The model under review builds one solid part; all positions refer to its coordinate system, in mm. Round coordinates to 2 decimals unless told otherwise and drop trailing zeros. Order: outer loops, then holes, each group sorted by start corner. A loop starts at its lowest first (then second) coordinate and runs counter-clockwise, first axis right, second up.
1) Consider section A-A (x = 119). Give the boundary of the cut face in (y, z), then the cut area to 3 significant figures.
2) To check wall thickness, follow L1, parallel to X at y = 7.5, z = 1177.1; L2, parallel to Y at x = 359.5, z = 911.5; L3, parallel to X at y = 13.5, z = -203.35. State the ranges of each line that lie inside material, in increasing order.
3) Consider section B-B (y = -71.5). Give the boundary of the cut face in (x, z).
4) Clearance check with flat-ended pins moving along their axes: P1, Ø7.5, axis at y = -766.5, z = 990.5, coming from the -X side; P2, Ø7.5, axis at y = 15, z = 550, coming from the +X side; P3, Ø21, axis at x = 352.21, z = -203.35, coming from the -Y side. State where each tip first meets the part, or that it passes through.
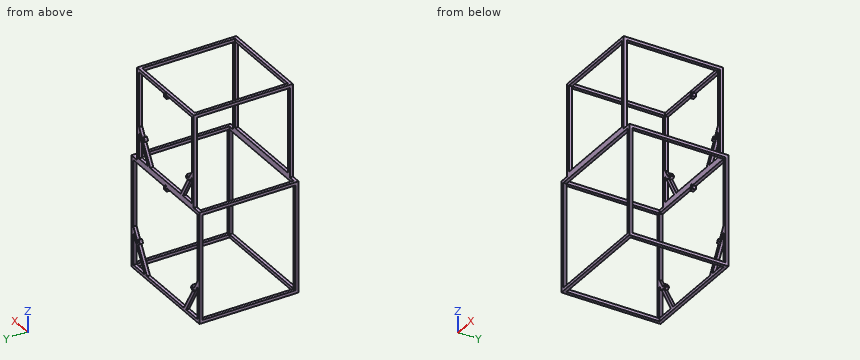
from build123d import *

# Parameters (mm, degrees)
BOSS_EXTRUDE1_DEPTH = 25
SKETCH2_R           = 6.5
CUT_EXTRUDE1_DEPTH  = 25
SKETCH3_W           = 25
SKETCH3_H           = 25
BOSS_EXTRUDE2_DEPTH = 750
SKETCH4_W           = 844.9
SKETCH4_H           = 844.9
SKETCH4_W_2         = 694.9
SKETCH4_H_2         = 694.9
BOSS_EXTRUDE3_DEPTH = 25


with BuildPart() as part:
    # Sketch1 → Boss-Extrude1 (new body)
    with BuildSketch(Plane(origin=(0, 0, 0), x_dir=(1, 0, 0), z_dir=(0, 1, 0))):
        Polygon((-447.45, -447.45), (-447.45, 447.45), (447.45, 447.45), (447.45, -447.45), (372.45, -447.45), (372.45, -1192.35), (-372.45, -1192.35), (-372.45, -447.45), align=None)
        Polygon((-422.45, 422.45), (-272.769134679, 422.45), (-422.45, 163.195136343), align=None, mode=Mode.SUBTRACT)
        Polygon((422.45, 113.195136343), (422.45, -422.45), (16, -422.45), (16, -394.45), (-16, -394.45), (-16, -422.45), (-422.45, -422.45), (-422.45, 113.195136343), (-373.852431829, 197.368593539), (-349.603720523, 183.368593539), (-333.603720523, 211.081406461), (-357.852431829, 225.081406461), (-243.901621219, 422.45), (243.901621219, 422.45), (357.852431829, 225.081406461), (333.603720523, 211.081406461), (349.603720523, 183.368593539), (373.852431829, 197.368593539), align=None, mode=Mode.SUBTRACT)
        Polygon((272.769134679, 422.45), (422.45, 163.195136343), (422.45, 422.45), align=None, mode=Mode.SUBTRACT)
        Polygon((-347.45, -472.45), (-229.467864489, -472.45), (-347.45, -676.80105309), align=None, mode=Mode.SUBTRACT)
        Polygon((229.467864489, -472.45), (347.45, -472.45), (347.45, -676.80105309), align=None, mode=Mode.SUBTRACT)
        Polygon((-200.60035103, -472.45), (200.60035103, -472.45), (292.900526545, -632.318593539), (268.651815239, -646.318593539), (284.651815239, -674.031406461), (308.900526545, -660.031406461), (347.45, -726.80105309), (347.45, -1167.35), (16, -1167.35), (16, -1139.35), (-16, -1139.35), (-16, -1167.35), (-347.45, -1167.35), (-347.45, -726.80105309), (-308.900526545, -660.031406461), (-284.651815239, -674.031406461), (-268.651815239, -646.318593539), (-292.900526545, -632.318593539), align=None, mode=Mode.SUBTRACT)
    extrude(amount=BOSS_EXTRUDE1_DEPTH)

    # Sketch2 → Cut-Extrude1 (cut)
    with BuildSketch(Plane(origin=(0, 25, 0), x_dir=(1, 0, 0), z_dir=(0, 1, 0))):
        with Locations(Location((0, -432.2, 0), (0, 0, 270))):
            Circle(SKETCH2_R)
        with Locations(Location((374.296179516, 216.1, 0), (0, 0, 270))):
            Circle(SKETCH2_R)
        with Locations(Location((352.212531719, 203.35, 0), (0, 0, 270))):
            Circle(SKETCH2_R)
        with Locations(Location((-374.296179516, 216.1, 0), (0, 0, 270))):
            Circle(SKETCH2_R)
        with Locations(Location((-352.212531719, 203.35, 0), (0, 0, 270))):
            Circle(SKETCH2_R)
        with Locations(Location((0, -1177.1, 0), (0, 0, 270))):
            Circle(SKETCH2_R)
        with Locations(Location((0, -1151.6, 0), (0, 0, 270))):
            Circle(SKETCH2_R)
        with Locations(Location((-309.344274232, -641.3, 0), (0, 0, 270))):
            Circle(SKETCH2_R)
        with Locations(Location((-287.260626435, -654.05, 0), (0, 0, 270))):
            Circle(SKETCH2_R)
        with Locations(Location((309.344274232, -641.3, 0), (0, 0, 270))):
            Circle(SKETCH2_R)
        with Locations(Location((287.260626435, -654.05, 0), (0, 0, 270))):
            Circle(SKETCH2_R)
        with Locations(Location((0, -406.7, 0), (0, 0, 270))):
            Circle(SKETCH2_R)
    extrude(amount=-CUT_EXTRUDE1_DEPTH, mode=Mode.SUBTRACT)

    # Sketch3 → Boss-Extrude2 (add)
    with BuildSketch(Plane.XZ):
        with Locations((-359.95, 1179.85)):
            Rectangle(SKETCH3_W, SKETCH3_H)
        with Locations((359.95, 1179.85)):
            Rectangle(SKETCH3_W, SKETCH3_H)
        with Locations((434.95, 434.95)):
            Rectangle(SKETCH3_W, SKETCH3_H)
        with Locations((-434.95, 434.95)):
            Rectangle(SKETCH3_W, SKETCH3_H)
        with Locations((434.95, -434.95)):
            Rectangle(SKETCH3_W, SKETCH3_H)
        with Locations((-434.95, -434.95)):
            Rectangle(SKETCH3_W, SKETCH3_H)
    extrude(amount=BOSS_EXTRUDE2_DEPTH)

    # Sketch4 → Boss-Extrude3 (add)
    with BuildSketch(Plane.XZ.offset(750)):
        Polygon((-372.45, 447.45), (-372.45, 1192.35), (372.45, 1192.35), (372.45, 447.45), (447.45, 447.45), (447.45, -447.45), (-447.45, -447.45), (-447.45, 447.45), align=None)
        Rectangle(SKETCH4_W, SKETCH4_H, mode=Mode.SUBTRACT)
        with Locations((0, 819.9)):
            Rectangle(SKETCH4_W_2, SKETCH4_H_2, mode=Mode.SUBTRACT)
    extrude(amount=BOSS_EXTRUDE3_DEPTH)


solid = part.part
Answer below:
1. outline: (-775, -447.45) - (-750, -447.45) - (-750, -422.45) - (-775, -422.45) - close; (-775, 422.45) - (-750, 422.45) - (-750, 472.45) - (-775, 472.45) - close; (-775, 1167.35) - (-750, 1167.35) - (-750, 1192.35) - (-775, 1192.35) - close; (0, -447.45) - (25, -447.45) - (25, -422.45) - (0, -422.45) - close; (0, 422.45) - (25, 422.45) - (25, 472.45) - (0, 472.45) - close; (0, 1167.35) - (25, 1167.35) - (25, 1192.35) - (0, 1192.35) - close
1. area: 5,000 mm2
2. L1: x = -372.45 to -6.5, 6.5 to 372.45
2. L2: y = -775 to -750, 0 to 25
2. L3: x = -447.45 to -422.45, -399.27 to -358.71, -345.71 to -338.07, 338.07 to 345.71, 358.71 to 399.27, 422.45 to 447.45
3. outline: (-447.45, -447.45) - (-422.45, -447.45) - (-422.45, -422.45) - (-447.45, -422.45) - close; (-447.45, 422.45) - (-422.45, 422.45) - (-422.45, 447.45) - (-447.45, 447.45) - close; (-372.45, 1167.35) - (-347.45, 1167.35) - (-347.45, 1192.35) - (-372.45, 1192.35) - close; (347.45, 1167.35) - (372.45, 1167.35) - (372.45, 1192.35) - (347.45, 1192.35) - close; (422.45, -447.45) - (447.45, -447.45) - (447.45, -422.45) - (422.45, -422.45) - close; (422.45, 422.45) - (447.45, 422.45) - (447.45, 447.45) - (422.45, 447.45) - close
4. P1: stops at x = -372.45
4. P2: stops at x = 372.45
4. P3: stops at y = 0
